The model under review builds one solid part; all positions refer to its coordinate system, in mm. A direction names the side the tool comes from. Coordinates: 2 decimals unless noted, no trailing zeros. Order: outer loops, then holes, each group sorted by start corner. A loop starts at its lowest first (then second) coordinate and runs counter-clockwise, first axis right, second up. Notation, with made-up numbers: (46.5, 8.5) - (58.5, 8.5) arc R22 ccw to (58.5, 27.5) - close; hole circle Ø7 at (55, 52). An arc over 180 degrees is marked (long way). Answer in a Markdown table with one row per item.
```python
from build123d import *

# Parameters (mm, degrees)
SKETCH1_R           = 2
BOSS_EXTRUDE1_DEPTH = 5
SKETCH2_W           = 0.1
SKETCH2_H           = 5
CUT_EXTRUDE1_DEPTH  = 3
SKETCH3_W           = 0.1
SKETCH3_H           = 5
CUT_EXTRUDE2_DEPTH  = 3
SKETCH5_W           = 5
SKETCH5_H           = 5
CUT_EXTRUDE3_DEPTH  = 3


with BuildPart() as part:
    # Sketch1 → Boss-Extrude1 (new body)
    with BuildSketch(Plane.XY):
        with BuildLine():
            Line((1, 0), (17, 0))
            ThreePointArc((17, 0), (24.071067812, -2.928932188), (27, -10))
            Line((27, -10), (27, -10.164726931))
            Line((27, -10.164726931), (27, -46.377180563))
            Line((27, -46.377180563), (26.694646109, -58.493944172))
            Line((26.694646109, -58.493944172), (26.694646109, -64.399649032))
            Line((26.694646109, -64.399649032), (26.694646109, -64.648499642))
            Line((26.694646109, -64.648499642), (45.291824906, -83.245678439))
            ThreePointArc((45.291824906, -83.245678439), (45.495822693, -83.59321769), (45.504515015, -83.996111065))
            Line((45.504515015, -83.996111065), (45.490365745, -84.055724665))
            ThreePointArc((45.490365745, -84.055724665), (45.211760066, -84.495661458), (44.721403846, -84.670922077))
            Line((44.721403846, -84.670922077), (36.743309345, -84.764807165))
            ThreePointArc((36.743309345, -84.764807165), (36.575585477, -84.749042296), (36.414881636, -84.698504168))
            ThreePointArc((36.414881636, -84.698504168), (34.774424803, -83.79382462), (33.33148975, -82.599051781))
            Line((33.33148975, -82.599051781), (21.037791859, -70.305353891))
            Line((21.037791859, -70.305353891), (16.801941123, -70.305353891))
            Line((16.801941123, -70.305353891), (1, -70.305353891))
            ThreePointArc((1, -70.305353891), (0.292893219, -70.012460672), (0, -69.305353891))
            Line((0, -69.305353891), (0, -64))
            ThreePointArc((0, -64), (0.292893219, -63.292893219), (1, -63))
            Line((1, -63), (10.539737479, -63))
            ThreePointArc((10.539737479, -63), (17.229153259, -60.229153259), (20, -53.539737479))
            Line((20, -53.539737479), (20, -16.460262521))
            ThreePointArc((20, -16.460262521), (17.229153259, -9.770846741), (10.539737479, -7))
            Line((10.539737479, -7), (1, -7))
            ThreePointArc((1, -7), (0.292893219, -6.707106781), (0, -6))
            Line((0, -6), (0, -1))
            ThreePointArc((0, -1), (0.292893219, -0.292893219), (1, 0))
        make_face()
        with Locations((35.887034264, -79.497742046)):
            Circle(SKETCH1_R, mode=Mode.SUBTRACT)
    extrude(amount=BOSS_EXTRUDE1_DEPTH)

    # Sketch2 → Cut-Extrude1 (cut)
    with BuildSketch(Plane(origin=(0, -63, 0), x_dir=(1, 0, 0), z_dir=(0, 1, 0))):
        with Locations((6.05, -2.5)):
            Rectangle(SKETCH2_W, SKETCH2_H)
    extrude(amount=-CUT_EXTRUDE1_DEPTH, mode=Mode.SUBTRACT)

    # Sketch3 → Cut-Extrude2 (cut)
    with BuildSketch(Plane.XZ.offset(7)):
        with Locations((6.05, 2.5)):
            Rectangle(SKETCH3_W, SKETCH3_H)
    extrude(amount=-CUT_EXTRUDE2_DEPTH, mode=Mode.SUBTRACT)

    # Sketch5 → Cut-Extrude3 (cut)
    with BuildSketch(Plane(origin=(17.315374744, -90.697945443, 0), x_dir=(0, 0, -1), z_dir=(0.18752569, -0.982259699, 0))):
        with Locations((-2.5, 23.878338891)):
            Rectangle(SKETCH5_W, SKETCH5_H)
    extrude(amount=-CUT_EXTRUDE3_DEPTH, mode=Mode.SUBTRACT)


solid = part.part
```
Item 1: We need section C-C, the plane y = -45. Write out the cut boundary in (x, z), then the cut area to 3 significant figures.
Check values:
| item | result |
|---|---|
| outline | (20, 0) - (27, 0) - (27, 5) - (20, 5) - close |
| area | 35.0 mm^2 |
Item 2: We need section A-A, the plane x = 8.5. Write out the cut boundary in (y, z), then the cut area to 3 significant figures.
Check values:
| item | result |
|---|---|
| outline | (-70.31, 0) - (-63, 0) - (-63, 5) - (-70.31, 5) - close; (-7, 0) - (0, 0) - (0, 5) - (-7, 5) - close |
| area | 71.5 mm^2 |
Item 3: Clearance check with flat-ended pins moving along their axes: pin 1 Ø1.5 at (y, z) = (-61.5, 1.5) entering from +X; pin 2 Ø3 at (y, z) = (-37, 2) entering from +X; pin 3 Ø2.5 at (x, z) = (12, 2) entering from -Y. State where each tip first meets the part, or that it passes through.
Check values:
| item | result |
|---|---|
| pin 1 | x = 26.69 |
| pin 2 | x = 27 |
| pin 3 | y = -70.31 |
Item 4: We need section B-B, the plane x = 14. Write out the cut boundary in (y, z).
Check values:
| item | result |
|---|---|
| outline | (-70.31, 0) - (-62.34, 0) - (-62.34, 5) - (-70.31, 5) - close; (-7.66, 0) - (0, 0) - (0, 5) - (-7.66, 5) - close |
Item 5: To check wall thickness, follow line 1 (Y direction, x = 10, z = 2.15); line 2 (Y direction, x = 14.5, z = 2.7); line 3 (X direction, y = -22.5, z = 1.9). State the ranges of each line that lie inside material, in increasing order. Write a range as from..to.
Check values:
| item | result |
|---|---|
| line 1 | -70.31..-63, -7..0 |
| line 2 | -70.31..-62.13, -7.87..0 |
| line 3 | 20..27 |
Item 6: Tool access review of faces 1 (the face through (11, -70.305, 2)), 2 (the face through (3, -63, 2)), 3 (the face through (27, -28, 2)): name each direction out of +Z, -Z, +X, -X, +Y, -Y from which nothing blocks a thin tool from reaching the whole face with its end or side.
Check values:
| item | result |
|---|---|
| face 1 | +Z, -Z, -X, -Y |
| face 2 | +Z, -Z, -X |
| face 3 | +Z, -Z, +X, +Y |
Item 7: We need section D-D, the plane x = 29.5. Write out the cut boundary in (y, z).
Check values:
| item | result |
|---|---|
| outline | (-78.77, 0) - (-67.45, 0) - (-67.45, 5) - (-78.77, 5) - close |
